Autodesk Fusion 360 part; units mm, degrees
sketch "Esquisse1" plane through (0, 0, 0) normal (0, 1, 0) x (1, 0, 0)
  line L0 (0, 0) -> (120, 0)
  line L1 (120, 0) -> (120, -100)
  line L2 (120, -100) -> (0, -100)
  line L3 (0, -100) -> (0, 0)
  line L4 (0, 0) -> (37.2, 0)
  line L5 (37.2, 0) -> (37.2, -32.2)
  line L6 (37.2, -32.2) -> (0, -32.2)
  line L7 (0, -32.2) -> (0, 0)
  line L8 (37.2, -32.2) -> (20.4, -32.2)
  line L9 (37.2, -7.4) -> (37.2, -32.2)
  line L10 (20.4, -32.2) -> (37.2, -7.4)
  line L11 (120, -100) -> (20.4, -32.2)
  line L12 (20.4, -32.2) -> (37.256, -7.4381)
  line L13 (37.256, -7.4381) -> (136.856, -75.2381)
  line L14 (136.856, -75.2381) -> (120, -100)
  line L15 (120, -100) -> (120, 0)
  line L16 (120, 0) -> (160, 0)
  line L17 (160, 0) -> (160, -100)
  line L18 (160, -100) -> (120, -100)
  line L19 (37.2, -7.4) -> (37.2, 0)
  line L20 (37.2, 0) -> (160, 0)
  line L21 (160, 0) -> (160, -7.4)
  line L22 (160, -7.4) -> (37.2, -7.4)
  line L23 (160, -7.4) -> (160, -100)
  line L24 (160, -100) -> (120, -100)
  line L25 (120, -100) -> (120, -7.4)
  line L26 (120, -7.4) -> (160, -7.4)
  dimension "d1" = 120
  dimension "d2" = 100
  dimension "d3" = 37.2
  dimension "d4" = 32.2
  dimension "d11" = 16.8
  dimension "d12" = 24.8
  dimension "d19" = 40
extrude "Extrusion3" add sketch "Esquisse1" along normal blind 200 contours L0 L3 L4 L5 L6 L7 L10 L19 | L0 L1 L5 L15 L19 L20 L22 | L1 L15 L16 L17 L20 L21 L22 L26 | L5 L6 L8 L9 L12 | L1 L5 L6 L8 L9 L11 L12 L13 L15 L25 | L1 L13 L14 L15 L17 L18 L22 L23 L24 L25 L26 | L1 L13 L14 L15 L25
extrude "Extrusion4" add sketch "Esquisse1" along normal blind 100 contours L0 L1 L5 L15 L19 L20 L22 | L2 L3 L6 L11 | L1 L15 L16 L17 L20 L21 L22 L26 | L1 L5 L9 L12 L13 L15 L22 L25 | L1 L13 L14 L15 L17 L18 L22 L23 L24 L25 L26
mirror "Symétrie miroir2" about plane through (0, 200, 0) normal (0, 1, 0) of bodies 1 merged
sketch "Esquisse3" plane through (-8.5188, 0, 12.5143) normal (-0.5627, 0, 0.8266) x (0, -1, 0)
  line L0 (-100, 34.9832) -> (-100, 155.4697)
  line L1 (-100, 155.4697) -> (-300, 155.4697)
  line L2 (-300, 155.4697) -> (-300, 34.9832)
  line L3 (-300, 34.9832) -> (-100, 34.9832)
  line L4 (-277.5, 138.4697) -> (-122.5, 138.4697)
  line L5 (-122.5, 138.4697) -> (-122.5, 52.4697)
  line L6 (-122.5, 52.4697) -> (-277.5, 52.4697)
  line L7 (-277.5, 52.4697) -> (-277.5, 138.4697)
  line L8 (-277.5, 138.4697) -> (-122.5, 52.4697) construction
  line L9 (-122.5, 138.4697) -> (-277.5, 52.4697) construction
  point P0 (-200, 95.4697)
  dimension "d22" = 155
  dimension "d23" = 86
  dimension "d24" = 22.5
  dimension "d25" = 17
extrude "Extrusion6" cut sketch "Esquisse3" against normal blind 2 contours L4 L5 L6 L7
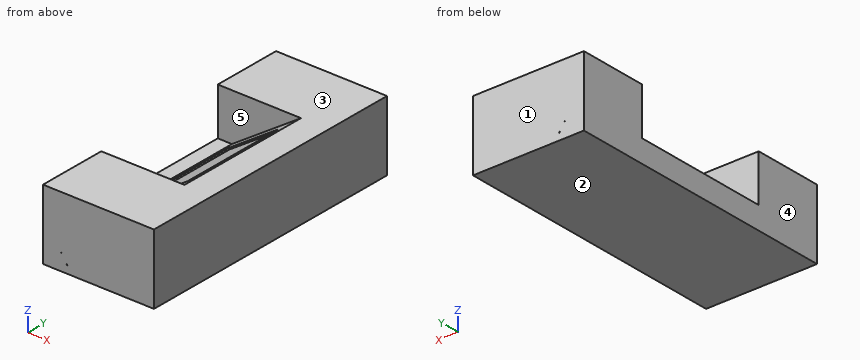
Geometry: final body of the model. Coordinates: model frame, mm. Face numbers are marked on the shaded views. A direction names the side the tool comes from. Round coordinates to 2 decimals unless told otherwise and drop trailing zeros. Order: outer loops, then holes, each group sorted by start corner. A loop starts at its lowest first (then second) coordinate and runs counter-clockwise, first axis right, second up. Notation, with made-up numbers: (88, 56) - (97, 56) arc R32 cw to (97, 88) - close; hole circle Ø4 at (-7, 69.25). An arc over 180 degrees is marked (long way). Use CSV: the item, a comma, the result in double quotes. Start each with the question number.
Q1. Section query C-C (x = 102). Return loops of the section in (y, z), and give its area (3 significant figures).
Q2. First-contact query: pin 1 (25 mm diameter, centred on x = 69, y = 155.5, fed in from +Z); pin 2 (12 mm diameter, centred on y = 120, z = 76.5, fed in from -X); pin 3 (12 mm diameter, centred on y = 195.5, z = 85.5, fed in from -X); pin 4 (12 mm diameter, centred on x = 123, y = 76, fed in from -Z). Flat tips, straight axial feed; report the tip coordinate or a pass-through.
Q3. Section query B-B (z = 11.5). Return loops of the section in (x, y).
Q4. Access query for the marked faces 4 and 5. Directions: +Z, -Z, +X, -X, +Y, -Y. A direction counts if a zero-diameter tool reaches every point of the face in a straight line with its end or side. Return the directions, or none.
Q5. Material intervals for line 1 along Y through (x, z) = (109.5, 40); line 2 along Z through (x, y) = (49, 168); line 3 along X through (y, z) = (192.5, 61.5), sorted ascending. Write a range as from..to.
Q6. Mould query, pull axis Z, two halves, no side actions, for the marked faces 1, 2 and 3. Classes: +Z half, -Z half, draft (parallel to the pull), parting line (faces both ways), or undercut.
Q7. Section query D-D (z = 78). Return loops of the section in (x, y), and give its area (3 significant figures).
Result set:
1,outline,"(0, 0) - (400, 0) - (400, 100) - (300, 100) - (300, 87.75) - (277.5, 87.75) - (277.5, 85.33) - (122.5, 85.33) - (122.5, 87.75) - (100, 87.75) - (100, 100) - (0, 100) - close; hole (100, 7.4) - (300, 7.4) - (300, 51.51) - (100, 51.51) - close"
1,area,"28,400 mm2"
2,pin 1,"stops at z = 71.37"
2,pin 2,"stops at x = 76.66"
2,pin 3,"stops at x = 93.44"
2,pin 4,"stops at z = 0"
3,outline,"(0, 0) - (34.42, 0) - (34.42, 400) - (0, 400) - close; (34.49, 0) - (160, 0) - (160, 400) - (34.49, 400) - close; hole (43.22, 100) - (120, 100) - (120, 300) - (43.22, 300) - close"
4,face 4,"+Z, -Z, -X, +Y, -Y"
4,face 5,"+Z, -X"
5,line 1,"y = 0..100, 300..400"
5,line 2,"z = 0..7.4, 15.43..49.25"
5,line 3,"x = 66.99..116.67, 120..160"
6,face 1,"draft"
6,face 2,"-Z half"
6,face 3,"+Z half"
7,outline,"(0, 0) - (160, 0) - (160, 400) - (0, 400) - (0, 300) - (87.68, 300) - (87.68, 277.5) - (91.23, 277.5) - (91.23, 122.5) - (87.68, 122.5) - (87.68, 100) - (0, 100) - close"
7,area,"45,900 mm2"
